Verification items for this drawing (mm, ordinates from the low corner). A direction names the side the tool comes from. Round coordinates to 2 decimals unless told otherwise and drop trailing zeros. Order: outer loops, then holes, each group sorted by start corner. A loop starts at its lowest first (then second) coordinate and runs counter-clockwise, first axis right, second up.
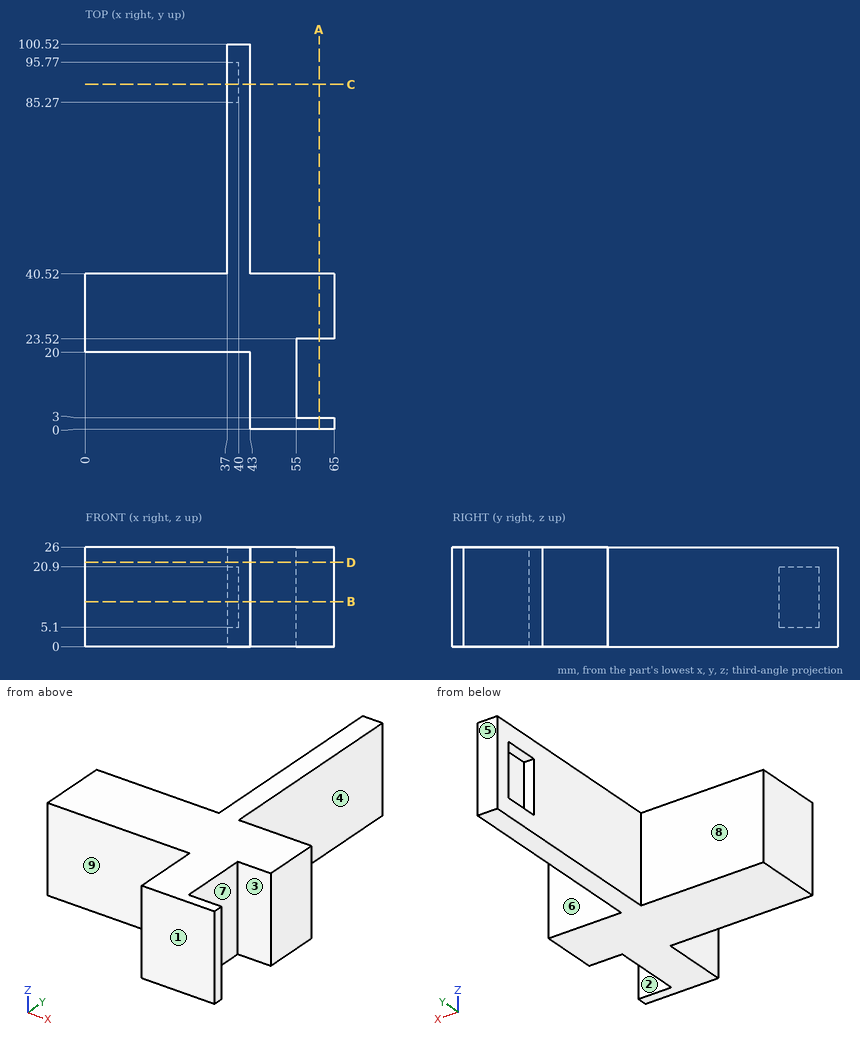
Item 1: Release check for a two-part mould opening along Y. For the marked faces 1, 2, 3 and 4 record: released by +Y, released by -Y, zero draft, split by the parting line, or undercut.
Answer:
face 1: released by -Y
face 2: undercut
face 3: undercut
face 4: zero draft
Item 2: Sectioned sample at B-B (z = 11.75). Record the cut outline in (x, y), and give its area (3 significant figures).
Answer:
outline: (0, 20) - (43, 20) - (43, 0) - (65, 0) - (65, 3) - (55, 3) - (55, 23.52) - (65, 23.52) - (65, 40.52) - (43, 40.52) - (43, 100.52) - (37, 100.52) - (37, 95.77) - (40, 95.77) - (40, 85.27) - (37, 85.27) - (37, 40.52) - (0, 40.52) - close
area: 1,900 mm2
Item 3: Sectioned sample at C-C (y = 90). Record the cut outline in (x, z).
Answer:
outline: (37, 0) - (43, 0) - (43, 26) - (37, 26) - (37, 20.9) - (40, 20.9) - (40, 5.1) - (37, 5.1) - close
Item 4: Access from +Z, -Z, +X, -X, +Y, -Y to the whole of each face (thin tool, end or side, straight path). Record for the marked faces 5, 6, 7, 8 and 9.
Answer:
face 5: +Z, -Z, +X, -X, +Y
face 6: +Z, -Z, +X, +Y
face 7: +Z, -Z, +X
face 8: +Z, -Z, -X, +Y
face 9: +Z, -Z, -X, -Y
Item 5: Sectioned sample at D-D (z = 22). Record the cut outline in (x, y).
Answer:
outline: (0, 20) - (43, 20) - (43, 0) - (65, 0) - (65, 3) - (55, 3) - (55, 23.52) - (65, 23.52) - (65, 40.52) - (43, 40.52) - (43, 100.52) - (37, 100.52) - (37, 40.52) - (0, 40.52) - close
Item 6: Sectioned sample at A-A (x = 61). Record the cut outline in (y, z), and give its area (3 significant figures).
Answer:
outline: (0, 0) - (3, 0) - (3, 26) - (0, 26) - close; (23.52, 0) - (40.52, 0) - (40.52, 26) - (23.52, 26) - close
area: 520 mm2
Item 7: Go/stop test with flat-tipped pins: P1, Ø1, axis at x = 33, z = 17.5, coming from the +Y side; P2, Ø2.5, axis at x = 38.5, z = 17, coming from the -Y side; P3, Ø8, axis at y = 67, z = 15, coming from the -X side; P4, Ø12, axis at x = 40, z = 13, coming from the -Y side. Record where each tip stops, or that it passes through.
Answer:
P1: stops at y = 40.52
P2: stops at y = 20
P3: stops at x = 37
P4: stops at y = 0
Item 8: Scan lines: line 1 along Y through (x, z) = (57, 8.75); line 2 along Y through (x, z) = (39.5, 16.5); line 3 along X through (y, z) = (86, 18). Record each from-to range of solid material in increasing order.
Answer:
line 1: y = 0 to 3, 23.52 to 40.52
line 2: y = 20 to 85.27, 95.77 to 100.52
line 3: x = 40 to 43
